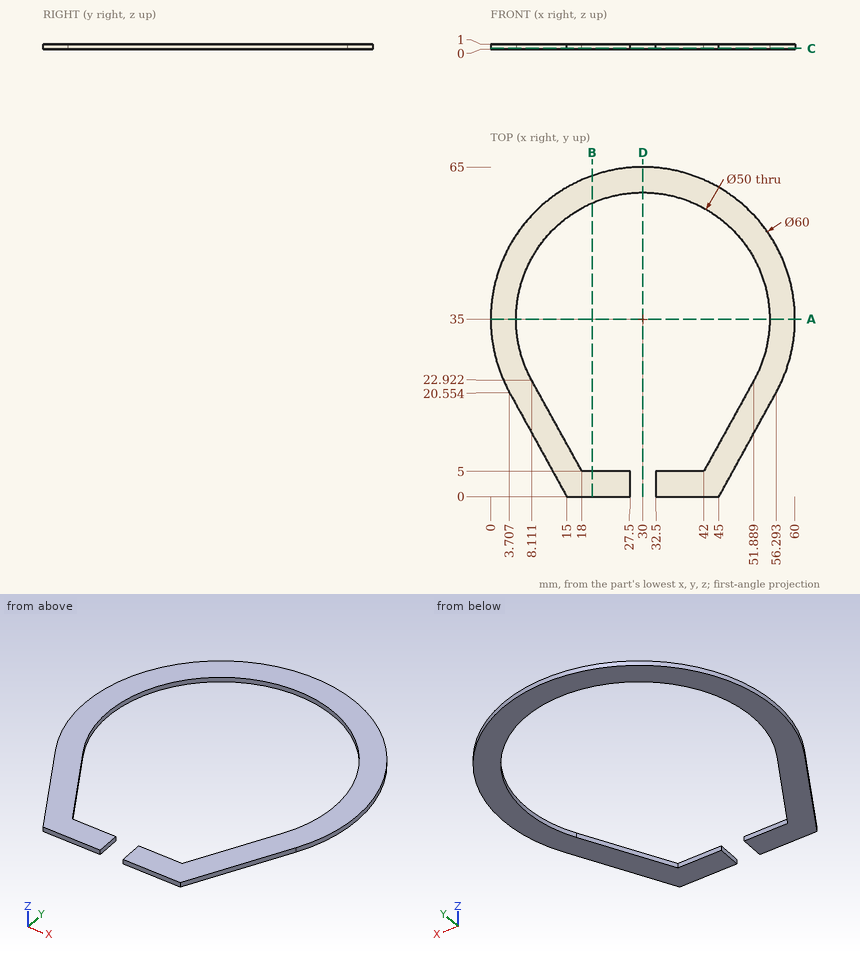
Verification items for this drawing (mm, ordinates from the low corner). Give positions to 0.01 mm unless a question says otherwise; leave off trailing zeros. Write each loop counter-clockwise with the first axis right and the second up, starting at its lowest first coordinate (ties: lowest second). Pieces come first, ordered by that corner, then holes. Notation, with made-up numbers: (12, 37) - (44, 37) arc R31 cw to (44, 66) - close; hole circle Ø9 at (17.5, -15). An arc over 180 degrees is marked (long way). Answer as CSV lines item,"result". Start each with the question number.
1. Sectioned sample at A-A (y = 35). Record the boundary of the cut face in (x, z), then the cut area to 3 significant figures.
2. Thickness scan on line 1 (X direction, y = 35, z = 0.6); line 2 (Y direction, x = 30, z = 0.5); line 3 (Y direction, x = 24, z = 0.1). Record the ranges inside material, lowest first.
3. Sectioned sample at C-C (z = 0.15). Record the boundary of the cut face in (x, y).
4. Depth check by flat-ended pin: pin 1 (0.5 mm diameter, centred on y = 2, z = 0.5, fed in from +X). Enter the tip coordinate at first touch or a pass-through.
5. Sectioned sample at D-D (x = 30). Record the boundary of the cut face in (y, z).
6. Sectioned sample at B-B (x = 20). Record the boundary of the cut face in (y, z), then the cut area to 3 significant figures.
Derived:
1,outline,"(0, 0) - (5, 0) - (5, 1) - (0, 1) - close; (55, 0) - (60, 0) - (60, 1) - (55, 1) - close"
1,area,"10.0 mm²"
2,line 1,"0 to 5, 55 to 60"
2,line 2,"60 to 65"
2,line 3,"0 to 5, 59.27 to 64.39"
3,outline,"(3.71, 20.55) - (15, 0) - (27.5, 0) - (27.5, 5) - (18, 5) - (8.11, 22.92) arc R25 cw (long way) to (51.89, 22.92) - (42, 5) - (32.5, 5) - (32.5, 0) - (45, 0) - (56.29, 20.55) arc R30 ccw (long way) to start"
4,pin 1,"x = 46.24"
5,outline,"(60, 0) - (65, 0) - (65, 1) - (60, 1) - close"
6,outline,"(0, 0) - (5, 0) - (5, 1) - (0, 1) - close; (57.91, 0) - (63.28, 0) - (63.28, 1) - (57.91, 1) - close"
6,area,"10.4 mm²"
